Input: part model. Units: mm. Frame: model coordinates. Coordinates: 2 decimals unless noted, no trailing zeros. Order: outer loops, then holes, each group sorted by start corner. A loop starts at its lowest first (then second) coordinate and runs counter-clockwise, first axis right, second up. Notation, with made-up numbers: (1, 27.25) - (38, 27.25) arc R26 ccw to (38, 55.25) - close; hole circle Ø6 at (67.5, 73). An arc over 180 degrees is marked (long way). One line per question, with ' | ' between items.
from build123d import *

# Parameters (mm, degrees)
SALIENTE_EXTRUIR1_DEPTH = 15
CROQUIS2_W              = 25
CROQUIS2_H              = 15
CORTAR_EXTRUIR1_DEPTH   = 21.55
REDONDEO2_R             = 10
CROQUIS3_W              = 40
CROQUIS3_H              = 19
CROQUIS3_H_2            = 12
CORTAR_EXTRUIR2_DEPTH   = 15


with BuildPart() as part:
    # Croquis1 → Saliente-Extruir1 (new, symmetric)
    with BuildSketch(Plane(origin=(0, 0, 0), x_dir=(1, 0, 0), z_dir=(0, 1, 0))):
        Polygon((15, 0), (160.588093706, 400), (110.588093706, 400), (-15, 0), align=None)
    extrude(amount=SALIENTE_EXTRUIR1_DEPTH, both=True)

    # Croquis2 → Cortar-Extruir1 (cut)
    with BuildSketch(Plane(origin=(0, 0, -400), x_dir=(-1, 0, 0), z_dir=(0, 0, -1))):
        with Locations((-148.088093706, 0)):
            Rectangle(CROQUIS2_W, CROQUIS2_H)
    extrude(amount=-CORTAR_EXTRUIR1_DEPTH, mode=Mode.SUBTRACT)

    # Redondeo2
    redondeo2_edges = [part.edges().sort_by_distance(p)[0] for p in [
        (110.588093706, 0, -400),
    ]]
    fillet(redondeo2_edges, radius=REDONDEO2_R)

    # Croquis3 → Cortar-Extruir2 (cut)
    with BuildSketch(Plane(origin=(0, 15, 0), x_dir=(1, 0, 0), z_dir=(0, 1, 0))):
        with Locations((131.470474965, 320)):
            Rectangle(CROQUIS3_W, CROQUIS3_H)
        with Locations((53.580844832, 106)):
            Rectangle(CROQUIS3_W, CROQUIS3_H_2)
    extrude(amount=-CORTAR_EXTRUIR2_DEPTH, mode=Mode.SUBTRACT)


solid = part.part
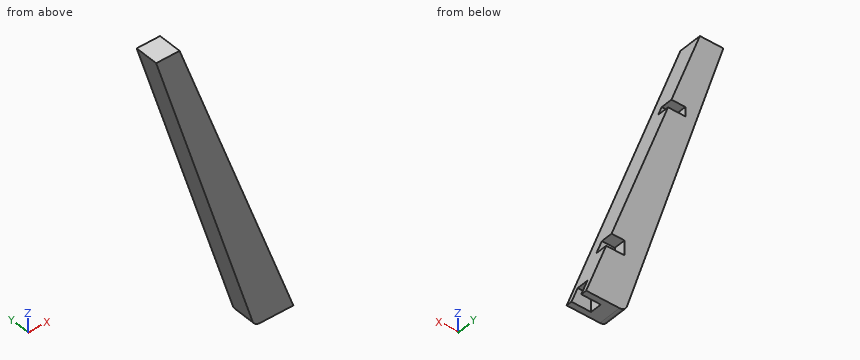
Item 1: Contact query for flat-ended pins moving along their axis: P1, Ø12, axis at y = 3, z = -392, coming from the +X side; P2, Ø6, axis at y = 5.5, z = -147, coming from the +X side; P3, Ø1, axis at x = 111.5, y = -8.5, coming from the -Z side. Output: stop coordinate, or through.
Data:
P1: x = 159.12 | P2: x = 69.6 | P3: z = -398.05
Item 2: Section C-C on z = -185. Return the cut outline in (x, y), and give its area (3 significant figures).
Data:
outline: (43.08, -15) - (82.33, -15) - (82.33, 15) - (43.08, 15) - close | area: 1,180 mm^2
Item 3: Section B-B on z = -324.5. Return the cut outline in (x, y).
Data:
outline: (86.88, -15) - (133.11, -15) - (133.11, 0) - (111.47, 0) - (111.47, 15) - (86.88, 15) - close
Item 4: Ray query, line 1 (Z direction, x = 133.5, y = 12.75); line 2 (X direction, y = 3.5, z = -297.5); line 3 (X direction, y = -6.5, z = -265). Return the intervals inside material, ascending.
Data:
line 1: -400 to -329.5 | line 2: 78.41 to 123.28 | line 3: 68.2 to 111.45
Item 5: Section D-D on x = 21.5. Return the cut outline in (y, z).
Data:
outline: (-15, -116.25) - (15, -116.25) - (15, -17.86) - (-15, -17.86) - close
Item 6: Section A-A on x = 141. Return the cut outline in (y, z).
Data:
outline: (-15, -400) - (-7.5, -400) - (-7.5, -378.45) - (7.5, -378.45) - (7.5, -400) - (15, -400) - (15, -346.18) - (-15, -346.18) - close
